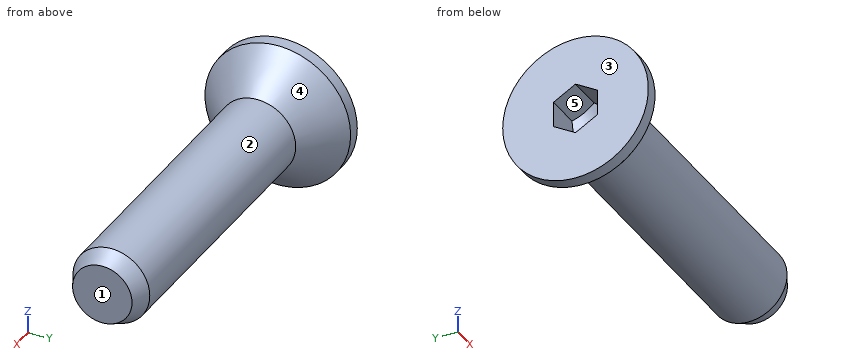
Autodesk Inventor part; units mm, degrees
ref_plane "Work Plane1" through (104.775, 0, 0) normal (0, 0, -1) x (1, 0, 0)
ref_plane "YZ Plane" through (0, 0, 0) normal (1, 0, 0) x (0, 1, 0)
ref_plane "XZ Plane" through (0, 0, 0) normal (0, 1, 0) x (-1, 0, 0)
sketch "Sketch1" plane through (0, 0, 0) normal (0, 0, 1) x (1, 0, 0)
  line L0 (19.05, 0) -> (19.05, 2.0828)
  line L1 (19.05, 2.0828) -> (4.8293, 2.0828)
  line L2 (4.8293, 2.0828) -> (2.8448, 2.0828)
  line L3 (0, 3.9497) -> (0, 1.3785)
  line L4 (0, 1.3785) -> (1.9304, 1.3785)
  line L5 (1.9304, 1.3785) -> (2.7263, 0)
  line L6 (2.7263, 0) -> (19.05, 0)
  line L7 (0, 3.9497) -> (0.6972, 3.9497)
  line L8 (0.6972, 3.9497) -> (2.8448, 2.0828)
  line L9 (2.8448, 2.0828) -> (2.8448, 2.0828)
  line L10 (4.8293, 2.0828) -> (2.8448, 2.0828) construction
  line L11 (2.8448, 2.0828) -> (2.8448, 2.0828)
  line L12 (-3.81, 0) -> (22.86, 0)
  line L13 (0, -0.7899) -> (0, 4.7396)
  dimension "d0" = 19.05
  dimension "d1" = 14.2207
  dimension "d2" = 1.9304
  dimension "d3" = 4.1656
  dimension "d6" = 2.8448
  dimension "d7" = 41
  dimension "d8" = 2.757
  dimension "d9" = 60
  dimension "d10" = 7.8994
  dimension "d11" = 4.1656
  dimension "d12" = 1.9845
revolve "Body" add sketch "Sketch1" angle 360 about axis through (2.7263, 0, 0) along (1, 0, 0) contours L6 L5 L4 L3 L7 L8 L2 L1 L0
sketch "Sketch2" plane through (0, 0, 0) normal (-1, 0, 0) x (0, 0, 1)
  circle A0 centre (0, 0) radius 1.3785
  line L0 (0, -5.5296) -> (0, 5.5296)
  line L1 (-5.5296, 0) -> (5.5296, 0)
  line L2 (1.3785, 0) -> (0.6892, -1.1938)
  line L3 (0.6892, -1.1938) -> (-0.6892, -1.1938)
  line L4 (-0.6892, -1.1938) -> (-1.3785, 0)
  line L5 (-1.3785, 0) -> (-0.6892, 1.1938)
  line L6 (-0.6892, 1.1938) -> (0.6892, 1.1938)
  line L7 (0.6892, 1.1938) -> (1.3785, 0)
  point P0 (0, 1.3785)
extrude "Slot" add sketch "Sketch2" against normal up to next contours L7 A0 | A0 L2 | L6 L0 A0 | A0 L0 L3 | L0 L6 A0 | A0 L3 L0 | L4 A0 | A0 L5
thread "Thread"
chamfer "Chamfer1" distance 0.4724 distance2 0.9449 1 edges at (19.05, -2.0828, 0) measured on face at (19.05, 0.3944, 0.7269)
ref_plane "Work Plane1" through (104.775, 0, 0) normal (0, 0, -1) x (1, 0, 0)
equation "\"d15\" = GEL"
equation "\"d17\" = -0.5 * SPD + 0.5 * GD"
equation "\"d18\" = GUL"
equation "\"d0\" = NLG"
equation "\"d1\" = GEL"
equation "\"d2\" = INTI"
equation "\"d3\" = GD"
equation "\"d6\" = KOH"
equation "\"d7\" = 0.5 * SEWI"
equation "\"d8\" = 1.1547 * SW"
equation "\"d10\" = KOD"
equation "\"d11\" = BDM"
equation "\"d12\" = GAL"
equation "\"NLG\" = 19.05"
equation "\"INTI\" = 1.9304"
equation "\"GEL\" = 14.2207"
equation "\"GAL\" = 1.9845"
equation "\"KOH\" = 2.8448"
equation "\"KOD\" = 7.8994"
equation "\"GUL\" = 0.94488"
equation "\"SPD\" = 3.22072"
equation "\"BDM\" = NND"
equation "\"GD\" = NND"
equation "\"SEWI\" = 82deg"
equation "\"SW\" = 2.3876"
equation "\"TOA\" = 30deg"
equation "\"GD1\" = SPD"
equation "\"THREADDIA\" = 4.1656"
equation "\"HHPTC\" = 0.79375"
equation "\"NND\" = 4.1656"
equation "\"E0\" = 1.155 * SW"
properties part number "ANSI B18.3 - 8-32 UNC x 0.75" material "Steel, Mild"
Source: CAD feature listing. Evaluate the final solid. Frame: model axes, mm. Face numbers are marked on the shaded views. A direction names the side the tool comes from. Give positions to 0.01 mm unless a question says otherwise; leave off trailing zeros. Order: outer loops, then holes, each group sorted by start corner. A loop starts at its lowest first (then second) coordinate and runs counter-clockwise, first axis right, second up. Notation, with made-up numbers: (79.25, 2) -> (104.25, 2) arc R17 ccw to (104.25, 22) -> close; hole circle Ø6 at (-31, 54). An arc over 180 degrees is marked (long way). Use a Markdown table: item, result.
Q1. Access query for the marked faces 1 and 2. Directions: +Z, -Z, +X, -X, +Y, -Y. A direction counts if a zero-diameter tool reaches every point of the face in a straight line with its end or side. Return the directions, or none.
A:
| item | result |
|---|---|
| face 1 | +Z, -Z, +X, +Y, -Y |
| face 2 | +X |
Q2. First-contact query: P1, Ø3, axis at x = 8, z = -1.5, coming from the +Y side; P2, Ø1.1, axis at x = 1.5, z = 0, coming from the +Y side. Flat tips, straight axial feed; report the tip coordinate or a pass-through.
A:
| item | result |
|---|---|
| P1 | y = 2.08 |
| P2 | y = 3.73 |
Q3. Pull-direction query (Z, two-part tool) for the marked faces 3, 4 and 5; classes: +Z half, -Z half, draft (parallel to the pull), parting line (faces both ways), or undercut.
A:
| item | result |
|---|---|
| face 3 | draft |
| face 4 | parting line |
| face 5 | undercut |
Q4. Section A-A (x = 8). Return the cut outline in (y, z).
A:
| item | result |
|---|---|
| outline | circle Ø4.17 at (0, 0) |
Q5. Material intervals for line 1 (Z direction, x = 5.25, y = 0.25); line 2 (Z direction, x = 14.25, y = -0.75); line 3 (X direction, y = -0.5, z = 3), sorted ascending. Write a range as [from, to].
A:
| item | result |
|---|---|
| line 1 | [-2.07, 2.07] |
| line 2 | [-1.94, 1.94] |
| line 3 | [0, 1.74] |
